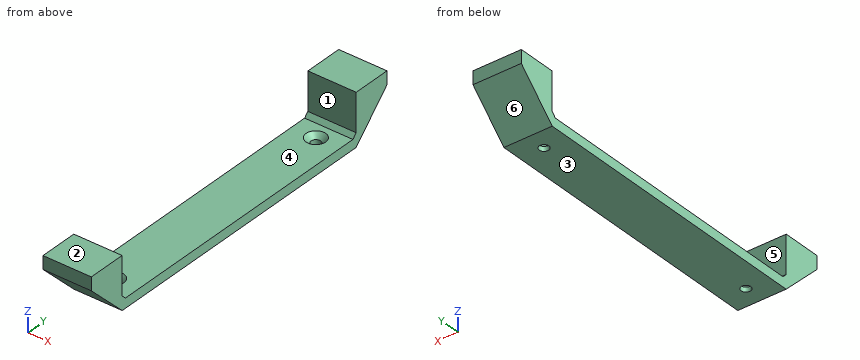
from build123d import *

# Parameters (mm, degrees)
PAD005_DEPTH        = 15
HOLE001_D           = 3
HOLE001_DEPTH       = 25
HOLE001_CSINK_D     = 6.1
HOLE001_CSINK_ANGLE = 90
HOLE_D              = 3
HOLE_DEPTH          = 25
HOLE_CSINK_D        = 6.1
HOLE_CSINK_ANGLE    = 90


with BuildPart() as part:
    # Sketch005 (on Face53 of Binder002) → Pad005 (new body)
    with BuildSketch(Plane(origin=(87.2, 0, 0), x_dir=(0, -1, 0), z_dir=(-1, 0, 0))):
        Polygon((-57.63, -4.868579), (-57.63, -0.81), (-45.63, -0.81), (-45.63, -12.625938), (-44.345938, -13.91), (0, -13.91), (0, -16.91), (-45.588579, -16.91), align=None)
    pad005 = extrude(amount=PAD005_DEPTH)

    # Mirrored: Pad005 across Sketch005 V_Axis
    add(pad005.mirror(Plane(origin=(87.2, 0, 0), x_dir=(-1, 0, 0), z_dir=(0, -1, 0))))

    # Hole001
    with Locations(Plane.XY.offset(-13.91)):
        with Locations((79.7, 39.345938), (79.7, -39.345938)):
            CounterSinkHole(HOLE001_D / 2, HOLE001_CSINK_D / 2, depth=HOLE001_DEPTH, counter_sink_angle=HOLE001_CSINK_ANGLE)

    # Hole
    with Locations(Plane.XY.offset(-13.91)):
        with Locations((79.7, 39.345938), (79.7, -39.345938)):
            CounterSinkHole(HOLE_D / 2, HOLE_CSINK_D / 2, depth=HOLE_DEPTH, counter_sink_angle=HOLE_CSINK_ANGLE)


with BuildPart() as part_1:
    # Body003 placement: moved
    add(part.part.moved(Location((-125, 0, 0))))


solid = part_1.part
CAD build for the part. Positions are in the model's coordinates, mm. Face numbers are marked on the shaded views. A direction names the side the tool comes from. Round coordinates to 2 decimals unless told otherwise and drop trailing zeros. Loops run counter-clockwise (first coordinate to the right, second up) from the corner with the lowest first, then second, coordinate; pieces in that order, holes last. Notation, with made-up numbers: (88.5, -13) - (97.5, -13) arc R23 cw to (97.5, 6) - close; hole circle Ø2 at (-33.5, -36.75). An arc over 180 degrees is marked (long way). Put each result on its own line as item: value.
1. 3-axis set-ups, long thin cutter, end or side, ignore diameter. For the marked faces 1 and 2: which of +Z, -Z, +X, -X, +Y, -Y reach the whole face in a straight line?
Geometry check:
face 1: +Z, +X, -X
face 2: +Z, +X, -X, +Y, -Y
2. Slice it at C-C on x = -38.75. List the corners of the cut face in (y, z).
Geometry check:
outline: (-57.63, -4.87) - (-45.59, -16.91) - (45.59, -16.91) - (57.63, -4.87) - (57.63, -0.81) - (45.63, -0.81) - (45.63, -12.63) - (44.35, -13.91) - (-44.35, -13.91) - (-45.63, -12.63) - (-45.63, -0.81) - (-57.63, -0.81) - close
3. Wall check: line 1 (Y direction, x = -45.3, z = -16.1); line 2 (Y direction, x = -45.3, z = -15.95); line 3 (Z direction, x = -40, y = 16). Give the ranges that are in metal, low to high.
Geometry check:
line 1: -46.4 to -40.85, -37.85 to 37.85, 40.85 to 46.4
line 2: -46.55 to -40.85, -37.85 to 37.85, 40.85 to 46.55
line 3: -16.91 to -13.91
4. Slice it at A-A on x = -45.3. List the corners of the cut face in (y, z).
Geometry check:
outline: (-57.63, -4.87) - (-45.59, -16.91) - (-40.85, -16.91) - (-40.85, -15.46) - (-42.4, -13.91) - (-44.35, -13.91) - (-45.63, -12.63) - (-45.63, -0.81) - (-57.63, -0.81) - close; (-37.85, -16.91) - (37.85, -16.91) - (37.85, -15.46) - (36.3, -13.91) - (-36.3, -13.91) - (-37.85, -15.46) - close; (40.85, -16.91) - (45.59, -16.91) - (57.63, -4.87) - (57.63, -0.81) - (45.63, -0.81) - (45.63, -12.63) - (44.35, -13.91) - (42.4, -13.91) - (40.85, -15.46) - close
5. Slice it at B-B on z = -8. List the corners of the cut face in (x, y), and give its area (3 significant figures).
Geometry check:
outline: (-52.8, -54.5) - (-37.8, -54.5) - (-37.8, -45.63) - (-52.8, -45.63) - close; (-52.8, 45.63) - (-37.8, 45.63) - (-37.8, 54.5) - (-52.8, 54.5) - close
area: 266 mm²
6. Two-plate mould, pull along Y, no slides. Class the marked faces 3, 4, 5 and 6: released by +Y, released by -Y, zero draft, split by the parting line, or undercut.
Geometry check:
face 3: zero draft
face 4: undercut
face 5: undercut
face 6: released by +Y
7. Slice it at D-D on y = -28. List the corners of the cut face in (x, z), and give its area (3 significant figures).
Geometry check:
outline: (-52.8, -16.91) - (-37.8, -16.91) - (-37.8, -13.91) - (-52.8, -13.91) - close
area: 45.0 mm²
8. Pin check, flat tips, straight feed: P1, Ø4, axis at x = -45, y = 2, coming from the +Z side; P2, Ø1, axis at x = -46, z = -8.5, coming from the +Y side; P3, Ø4, axis at x = -45, z = -12.5, coming from the -Y side. Stop position of each tip, or through.
Geometry check:
P1: z = -13.91
P2: y = 54.5
P3: y = -52
